Read the model definition and answer for the solid it produces. Units are mm, in the model's axes. Face numbers are marked on the shaded views. A direction names the side the tool comes from. Coordinates: 2 decimals unless noted, no trailing zeros. Write each loop counter-clockwise with the first axis right and the second up, starting at its lowest first coordinate (ties: lowest second). Pieces come first, ordered by that corner, then holes. Notation, with made-up numbers: (35.25, 58) - (90.25, 58) arc R24 ccw to (90.25, 89) - close; hole circle Ø2 at (-13, 52.5). An arc over 180 degrees is marked (long way). Use a Markdown table: item, result.
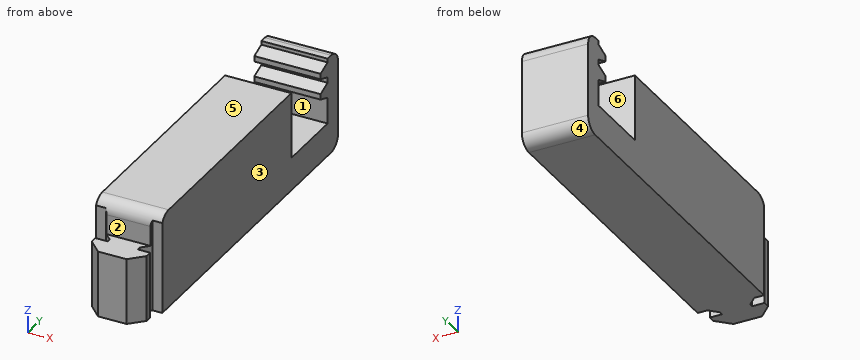
from build123d import *

# Parameters (mm, degrees)
BOSS_EXTRUDE1_DEPTH = 6.35
CUT_EXTRUDE1_DEPTH  = 13.7
CUT_EXTRUDE2_DEPTH  = 20.05
FILLET1_R           = 2.54
CUT_EXTRUDE3_DEPTH  = 20.05
SKETCH6_W           = 12.7
SKETCH6_H           = 0.396875
CUT_EXTRUDE4_DEPTH  = 13.7


with BuildPart() as part:
    # Sketch1 → Boss-Extrude1 (new body, symmetric)
    with BuildSketch(Plane(origin=(0, 0, 0), x_dir=(0, 0, -1), z_dir=(1, 0, 0))):
        Polygon((6.35, 0), (6.35, -6.096), (19.05, -6.096), (19.05, 63.754508), (12.7, 63.754508), (0, 63.754508), (0, 57.404508), (12.7, 57.404508), (12.7, 47.244508), (0, 47.244508), (0, 0), align=None)
    extrude(amount=BOSS_EXTRUDE1_DEPTH, both=True)

    # Sketch2 → Cut-Extrude1 (cut, through all)
    with BuildSketch(Plane(origin=(6.35, 0, 0), x_dir=(0, 0, -1), z_dir=(1, 0, 0))):
        with BuildLine():
            Line((12.7, 57.404508), (6.715252, 57.404508))
            Line((6.715252, 57.404508), (6.665278777, 57.267207698))
            ThreePointArc((6.665278777, 57.267207698), (6.572077823, 57.14574585), (6.426064417, 57.099708))
            Line((6.426064417, 57.099708), (5.934007978, 57.099708))
            ThreePointArc((5.934007978, 57.099708), (5.787994572, 57.14574585), (5.694793618, 57.267207698))
            Line((5.694793618, 57.267207698), (5.644820395, 57.404508))
            Line((5.644820395, 57.404508), (2.72542, 57.404508))
            Line((2.72542, 57.404508), (2.675446777, 57.267207698))
            ThreePointArc((2.675446777, 57.267207698), (2.582245823, 57.14574585), (2.436232417, 57.099708))
            Line((2.436232417, 57.099708), (1.944175978, 57.099708))
            ThreePointArc((1.944175978, 57.099708), (1.798162572, 57.14574585), (1.704961618, 57.267207698))
            Line((1.704961618, 57.267207698), (1.654988395, 57.404508))
            Line((1.654988395, 57.404508), (0, 57.404508))
            Line((0, 57.404508), (0, 47.244508))
            Line((0, 47.244508), (12.7, 47.244508))
            Line((12.7, 47.244508), (12.7, 57.404508))
        make_face()
        Polygon((2.72542, 57.404508), (5.644820395, 57.404508), (4.720336, 59.944508), (3.649904395, 59.944508), align=None)
        Polygon((0, 57.404508), (1.654988395, 57.404508), (0.730504, 59.944508), (0, 59.944508), align=None)
        Polygon((8.710168, 59.944508), (7.639736395, 59.944508), (6.715252, 57.404508), (12.7, 57.404508), (12.7, 59.944508), align=None)
    extrude(amount=-CUT_EXTRUDE1_DEPTH, mode=Mode.SUBTRACT)

    # Sketch3 → Cut-Extrude2 (cut, through all)
    with BuildSketch(Plane(origin=(0, 0, -19.05), x_dir=(-1, 0, 0), z_dir=(0, 0, -1))):
        Polygon((-6.35, -6.096), (-2.839339828, -6.1), (-5.5, -3.439339828), (-5.5, -1.8), (-3.125, -1.8), (-3.125, -1.455), (-4.58, 0), (-9.5, 0), align=None)
        Polygon((2.839339828, -6.1), (6.35, -6.096), (15.42, 0), (4.58, 0), (3.125, -1.455), (3.125, -1.8), (5.5, -1.8), (5.5, -3.439339828), align=None)
    extrude(amount=-CUT_EXTRUDE2_DEPTH, mode=Mode.SUBTRACT)

    # Fillet1
    fillet1_edges = [part.edges().sort_by_distance(p)[0] for p in [
        (0, 63.754508, 0),
        (0, 63.754508, -19.05),
        (0, 0, 0),
    ]]
    fillet(fillet1_edges, radius=FILLET1_R)

    # Sketch5 → Cut-Extrude3 (cut, through all)
    with BuildSketch(Plane(origin=(0, 0, -19.05), x_dir=(-1, 0, 0), z_dir=(0, 0, -1))):
        Polygon((6.35, 0), (4.58, 0), (3.125, -1.455), (3.125, -1.8), (5.5, -1.8), (5.5, -3.439339828), (2.843339828, -6.096), (-2.843339828, -6.096), (-5.5, -3.439339828), (-5.5, -1.8), (-3.125, -1.8), (-3.125, -1.455), (-4.58, 0), (-6.35, 0), (-6.35, 0.254), (-4.474789755, 0.254), (-2.871, -1.349789755), (-2.871, -2.054), (-5.246, -2.054), (-5.246, -3.334129583), (-2.738129583, -5.842), (2.738129583, -5.842), (5.246, -3.334129583), (5.246, -2.054), (2.871, -2.054), (2.871, -1.349789755), (4.474789755, 0.254), (6.35, 0.254), align=None)
    extrude(amount=-CUT_EXTRUDE3_DEPTH, mode=Mode.SUBTRACT)

    # Sketch6 → Cut-Extrude4 (cut, through all)
    with BuildSketch(Plane(origin=(6.35, 0, 0), x_dir=(0, 0, -1), z_dir=(1, 0, 0))):
        with Locations((6.35, 47.0460705)):
            Rectangle(SKETCH6_W, SKETCH6_H)
    extrude(amount=-CUT_EXTRUDE4_DEPTH, mode=Mode.SUBTRACT)


solid = part.part
(1) Straight lines are drawn through the part: L1, parallel to Y at x = -0.5, z = -7.75; L2, parallel to Y at x = -4.75, z = -12; L3, parallel to Y at x = -0.75, z = -6.25. For each, find the intervals that lie inside material, in ascending order.
Report:
| item | result |
|---|---|
| L1 | y = -5.84 to 46.85, 59.94 to 63.75 |
| L2 | y = -3.83 to -2.05, 0.25 to 46.85, 59.94 to 63.75 |
| L3 | y = 0 to 46.85, 57.4 to 63.75 |
(2) For the marked faces 1, 2 and 3, determine the directions among +Z, -Z, +X, -X, +Y, -Y from which every point of the face is accessible in a straight line to the end or side of a thin tool.
Report:
| item | result |
|---|---|
| face 1 | +X, -X |
| face 2 | +Z, +X, -X, -Y |
| face 3 | +Z, -Z, +X, +Y, -Y |
(3) The mould has two halves that part along Y. Classify the marked faces 4, 5 and 6: pulls with the +Y half, pulls with the -Y half, needs draft (parallel to the pull), parting line crosses it, or undercut.
Report:
| item | result |
|---|---|
| face 4 | pulls with the +Y half |
| face 5 | needs draft |
| face 6 | undercut |
(4) A cutting plane is placed at A-A, the plane z = -9. Write down the section's boundary in (x, y), and give its area (3 significant figures).
Report:
| item | result |
|---|---|
| outline | (-6.35, 0.25) - (-4.47, 0.25) - (-2.87, -1.35) - (-2.87, -2.05) - (-5.25, -2.05) - (-5.25, -3.33) - (-2.74, -5.84) - (2.74, -5.84) - (5.25, -3.33) - (5.25, -2.05) - (2.87, -2.05) - (2.87, -1.35) - (4.47, 0.25) - (6.35, 0.25) - (6.35, 46.85) - (-6.35, 46.85) - close; (-6.35, 59.94) - (6.35, 59.94) - (6.35, 63.75) - (-6.35, 63.75) - close |
| area | 689 mm² |
(5) A cutting plane is placed at B-B, the plane x = 0. Write down the section's boundary in (y, z), and give its area (3 significant figures).
Report:
| item | result |
|---|---|
| outline | (-5.84, -19.05) - (61.21, -19.05) arc R2.54 ccw to (63.75, -16.51) - (63.75, -2.54) arc R2.54 ccw to (61.21, 0) - (59.94, 0) - (59.94, -0.73) - (57.4, -1.65) - (57.4, -2.73) - (59.94, -3.65) - (59.94, -4.72) - (57.4, -5.64) - (57.4, -6.72) - (59.94, -7.64) - (59.94, -12.7) - (46.85, -12.7) - (46.85, 0) - (2.54, 0) arc R2.54 ccw to (0, -2.54) - (0, -6.35) - (-5.84, -6.35) - close |
| area | 1,130 mm² |
(6) A cutting plane is placed at C-C, the plane z = -14.75. Write down the section's boundary in (x, y), and give its area (3 significant figures).
Report:
| item | result |
|---|---|
| outline | (-6.35, 0.25) - (-4.47, 0.25) - (-2.87, -1.35) - (-2.87, -2.05) - (-5.25, -2.05) - (-5.25, -3.33) - (-2.74, -5.84) - (2.74, -5.84) - (5.25, -3.33) - (5.25, -2.05) - (2.87, -2.05) - (2.87, -1.35) - (4.47, 0.25) - (6.35, 0.25) - (6.35, 63.75) - (-6.35, 63.75) - close |
| area | 856 mm² |
(7) Each of these flat-tipped pins is pushed along its axis until it touches: P1, Ø0.9, axis at x = -3, z = -2, coming from the -Y side; P2, Ø3, axis at x = 2, y = -2, coming from the +Z side; P3, Ø4, axis at x = 2.5, y = 50, coming from the +Z side. Where does it stop, or does it pass through?
Report:
| item | result |
|---|---|
| P1 | stops at y = 0 |
| P2 | stops at z = -6.35 |
| P3 | stops at z = -12.7 |
(8) A cutting plane is placed at D-D, the plane y = 51. Write down the section's boundary in (x, z), and give its area (3 significant figures).
Report:
| item | result |
|---|---|
| outline | (-6.35, -19.05) - (6.35, -19.05) - (6.35, -12.7) - (-6.35, -12.7) - close |
| area | 80.6 mm² |
